from build123d import *

# Parameters (mm, degrees)
SKETCH1_R           = 1.75
BOSS_EXTRUDE1_DEPTH = 4


with BuildPart() as part:
    # Sketch1 → Boss-Extrude1 (new body)
    with BuildSketch(Plane.YZ):
        with BuildLine():
            Line((-0.31, 14.63), (0.31, 14.63))
            ThreePointArc((0.31, 14.63), (0.838273314, 13.383704325), (1.04, 12.04518576))
            ThreePointArc((1.04, 12.04518576), (1.578061664, 11.986568374), (2.112960617, 11.903927815))
            ThreePointArc((2.112960617, 11.903927815), (2.65424773, 13.144626757), (3.487085624, 14.211728743))
            Line((3.487085624, 14.211728743), (4.085959636, 14.051260935))
            ThreePointArc((4.085959636, 14.051260935), (4.273667417, 12.71070456), (4.122086336, 11.365584201))
            ThreePointArc((4.122086336, 11.365584201), (4.626642697, 11.169703548), (5.12192646, 10.951436862))
            ThreePointArc((5.12192646, 10.951436862), (5.965886177, 12.009764599), (7.046532125, 12.824951657))
            Line((7.046532125, 12.824951657), (7.583467875, 12.514951657))
            ThreePointArc((7.583467875, 12.514951657), (7.417818147, 11.171491285), (6.9232593, 9.911436862))
            ThreePointArc((6.9232593, 9.911436862), (7.359925677, 9.591641884), (7.781841479, 9.252623584))
            ThreePointArc((7.781841479, 9.252623584), (8.870959341, 10.05645683), (10.125769107, 10.564175311))
            Line((10.125769107, 10.564175311), (10.564175311, 10.125769107))
            ThreePointArc((10.564175311, 10.125769107), (10.05645683, 8.870959341), (9.252623584, 7.781841479))
            ThreePointArc((9.252623584, 7.781841479), (9.591641884, 7.359925677), (9.911436862, 6.9232593))
            ThreePointArc((9.911436862, 6.9232593), (11.171491285, 7.417818147), (12.514951657, 7.583467875))
            Line((12.514951657, 7.583467875), (12.824951657, 7.046532125))
            ThreePointArc((12.824951657, 7.046532125), (12.009764599, 5.965886177), (10.951436862, 5.12192646))
            ThreePointArc((10.951436862, 5.12192646), (11.194344337, 4.566700654), (11.409123542, 4))
            Line((11.409123542, 4), (30.75, 4))
            ThreePointArc((30.75, 4), (34.75, 0), (30.75, -4))
            Line((30.75, -4), (11.409123542, -4))
            ThreePointArc((11.409123542, -4), (1.642293391, -11.977936902), (-9.911436862, -6.9232593))
            ThreePointArc((-9.911436862, -6.9232593), (-11.171491285, -7.417818147), (-12.514951657, -7.583467875))
            Line((-12.514951657, -7.583467875), (-12.824951657, -7.046532125))
            ThreePointArc((-12.824951657, -7.046532125), (-12.009764599, -5.965886177), (-10.951436862, -5.12192646))
            ThreePointArc((-10.951436862, -5.12192646), (-11.169703548, -4.626642697), (-11.365584201, -4.122086336))
            ThreePointArc((-11.365584201, -4.122086336), (-12.71070456, -4.273667417), (-14.051260935, -4.085959636))
            Line((-14.051260935, -4.085959636), (-14.211728743, -3.487085624))
            ThreePointArc((-14.211728743, -3.487085624), (-13.144626757, -2.65424773), (-11.903927815, -2.112960617))
            ThreePointArc((-11.903927815, -2.112960617), (-11.986568374, -1.578061664), (-12.04518576, -1.04))
            ThreePointArc((-12.04518576, -1.04), (-13.383704325, -0.838273314), (-14.63, -0.31))
            Line((-14.63, -0.31), (-14.63, 0.31))
            ThreePointArc((-14.63, 0.31), (-13.383704325, 0.838273314), (-12.04518576, 1.04))
            ThreePointArc((-12.04518576, 1.04), (-11.986568374, 1.578061664), (-11.903927815, 2.112960617))
            ThreePointArc((-11.903927815, 2.112960617), (-13.144626757, 2.65424773), (-14.211728743, 3.487085624))
            Line((-14.211728743, 3.487085624), (-14.051260935, 4.085959636))
            ThreePointArc((-14.051260935, 4.085959636), (-12.71070456, 4.273667417), (-11.365584201, 4.122086336))
            ThreePointArc((-11.365584201, 4.122086336), (-11.169703548, 4.626642697), (-10.951436862, 5.12192646))
            ThreePointArc((-10.951436862, 5.12192646), (-12.009764599, 5.965886177), (-12.824951657, 7.046532125))
            Line((-12.824951657, 7.046532125), (-12.514951657, 7.583467875))
            ThreePointArc((-12.514951657, 7.583467875), (-11.171491285, 7.417818147), (-9.911436862, 6.9232593))
            ThreePointArc((-9.911436862, 6.9232593), (-9.591641884, 7.359925677), (-9.252623584, 7.781841479))
            ThreePointArc((-9.252623584, 7.781841479), (-10.05645683, 8.870959341), (-10.564175311, 10.125769107))
            Line((-10.564175311, 10.125769107), (-10.125769107, 10.564175311))
            ThreePointArc((-10.125769107, 10.564175311), (-8.870959341, 10.05645683), (-7.781841479, 9.252623584))
            ThreePointArc((-7.781841479, 9.252623584), (-7.359925677, 9.591641884), (-6.9232593, 9.911436862))
            ThreePointArc((-6.9232593, 9.911436862), (-7.417818147, 11.171491285), (-7.583467875, 12.514951657))
            Line((-7.583467875, 12.514951657), (-7.046532125, 12.824951657))
            ThreePointArc((-7.046532125, 12.824951657), (-5.965886177, 12.009764599), (-5.12192646, 10.951436862))
            ThreePointArc((-5.12192646, 10.951436862), (-4.626642697, 11.169703548), (-4.122086336, 11.365584201))
            ThreePointArc((-4.122086336, 11.365584201), (-4.273667417, 12.71070456), (-4.085959636, 14.051260935))
            Line((-4.085959636, 14.051260935), (-3.487085624, 14.211728743))
            ThreePointArc((-3.487085624, 14.211728743), (-2.65424773, 13.144626757), (-2.112960617, 11.903927815))
            ThreePointArc((-2.112960617, 11.903927815), (-1.578061664, 11.986568374), (-1.04, 12.04518576))
            ThreePointArc((-1.04, 12.04518576), (-0.838273314, 13.383704325), (-0.31, 14.63))
        make_face()
        with Locations(Location((0, 0, 0), (0, 0, 270))):
            Circle(SKETCH1_R, mode=Mode.SUBTRACT)
        with Locations(Location((30.75, 0, 0), (0, 0, 270))):
            Circle(SKETCH1_R, mode=Mode.SUBTRACT)
    extrude(amount=BOSS_EXTRUDE1_DEPTH)


solid = part.part
Can you work these out from the model? Positions are in its coordinate system, mm. A direction names the side the tool comes from. Coordinates: 2 decimals unless noted, no trailing zeros. Loops run counter-clockwise (first coordinate to the right, second up) from the corner with the lowest first, then second, coordinate; pieces in that order, holes last. Notation, with made-up numbers: (-23, 23.25) - (22, 23.25) arc R26 cw to (22, 61.25) - close; hole circle Ø11 at (1, -31). An arc over 180 degrees is marked (long way). Answer as a JSON object with one key per item and string values. Group by question number.
Item 1: On a 3-axis mill with a long thin cutter (end or side, diameter ignored), from which of +Z, -Z, +X, -X, +Y, -Y can I reach the whole of each face in a straight line? I mean faces 1 (the face through (1.972, -13.402, 0.833)), 2 (the face through (1.972, -11.153, -7.413)), 3 (the face through (1.972, 7.422, 11.19)). Say none if no direction works.
Item 2: If I drill on L1, parallel to Y at x = 2.25, z = 0; L2, parallel to Y at x = 1.15, z = 12.5; L3, parallel to Y at x = 0.4, z = 10, over which ranges is the centre line in solid material (lowest first)? Write a range as from..to.
Item 3: For pin 1 (2 mm diameter, centred on x = 0.5, y = -8, fed in from -Z); pin 2 (2 mm diameter, centred on y = 19.5, z = 6.5, fed in from +X); pin 3 (1.2 mm diameter, centred on x = 1.5, y = 24.5, fed in from +Z); pin 4 (1 mm diameter, centred on x = 1, z = 1, fed in from +Y), each with a flat end and sliding along its axis, tell me the tip position at first contact or that it passes through.
Item 4: If we mould it in two halves opening along Z, with no side actions, what happens to faces 4 (the face through (1.972, -10.047, 8.854)), 5 (the face through (0, 5, 1)), 6 (the face through (1.972, 1.571, 11.988)), 7 (the face through (1.972, -13.161, -2.664))? For each: released by +Z, released by -Z, zero draft, split by the parting line, or undercut.
Item 5: If we section it at A-A (x = 3.5): State how many separate pieces and enclosed holes the cut face has, plus the area to 3 significant figures.
Item 6: If we section it at B-B (y = 22): List the corners of the cut face in (x, z) for me, plus the area to 3 significant figures.
Returned:
{
 "1": {"face 1": "+X, -X, -Y", "face 2": "-Z, +X, -X", "face 3": "+X, -X"},
 "2": {"L1": "y = -14.63..-1.75, 1.75..29, 32.5..34.75", "L2": "y = -7.58..-6.55, -4.27..-2.33, -1.01..1.01, 2.33..4.27, 6.55..7.58", "L3": "y = -10.53..-8.77, -6.97..6.97, 8.77..10.53"},
 "3": {"pin 1": "stops at z = -9.86", "pin 2": "passes through", "pin 3": "stops at z = 4", "pin 4": "stops at y = 34.72"},
 "4": {"face 4": "undercut", "face 5": "zero draft", "face 6": "released by +Z", "face 7": "undercut"},
 "5": {"separate pieces": "1", "enclosed holes": "2", "area": "669 mm²"},
 "6": {"outline": "(0, -4) - (4, -4) - (4, 4) - (0, 4) - close", "area": "32.0 mm²"}
}
